Read the model definition and answer for the solid it produces. Units are mm, in the model's axes. Face numbers are marked on the shaded views. A direction names the side the tool comes from. Round coordinates to 2 decimals unless told otherwise and drop trailing zeros. Order: outer loops, then holes, each group sorted by start corner. A loop starts at its lowest first (then second) coordinate and runs counter-clockwise, first axis right, second up.
Autodesk Inventor part; units mm, degrees
ref_plane "YZ Plane" through (0, 0, 0) normal (1, 0, 0) x (0, 1, 0)
ref_plane "XZ Plane" through (0, 0, 0) normal (0, 1, 0) x (-1, 0, 0)
ref_plane "XY Plane" through (0, 0, 0) normal (0, 0, 1) x (1, 0, 0)
sketch "Sketch1" plane through (0, 0, 0) normal (0, 0, 1) x (1, 0, 0)
  circle A0 centre (0, 0) radius 42.5
  dimension "d0" = 85
extrude "Extrusion1" add sketch "Sketch1" along normal blind 5
sketch "Sketch2" plane through (0, 0, 5) normal (0, 0, 1) x (1, 0, 0)
  circle A0 centre (0, 0) radius 13
  dimension "d3" = 26
extrude "Extrusion2" add sketch "Sketch2" along normal blind 20
sketch "Sketch3" plane through (0, 0, 25) normal (0, 0, 1) x (1, 0, 0)
  circle A0 centre (0, 0) radius 42.5
  dimension "d6" = 85
extrude "Extrusion3" add sketch "Sketch3" along normal blind 5
sketch "Sketch4" plane through (0, 0, 0) normal (0, 0, -1) x (-1, 0, 0)
  circle A0 centre (0, 0) radius 11
  dimension "d9" = 22
extrude "Extrusion4" cut sketch "Sketch4" against normal through all
properties part number "wire_spool_holder"
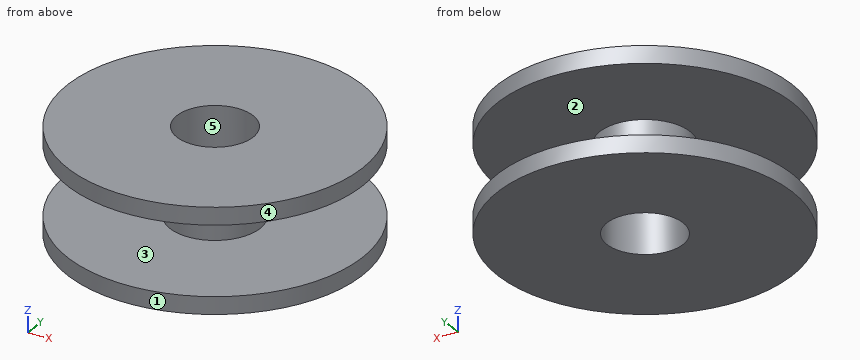
Q1. For the marked faces 1 and 2, determine the directions among +Z, -Z, +X, -X, +Y, -Y from which every point of the face is accessible in a straight line to the end or side of a thin tool.
Outcome:
face 1: +Z, -Z
face 2: none
Q2. A cutting plane is placed at A-A, the plane x = -25.5. Give the vertices of the cut face in (y, z).
Outcome:
outline: (-34, 0) - (34, 0) - (34, 5) - (-34, 5) - close; (-34, 25) - (34, 25) - (34, 30) - (-34, 30) - close
Q3. Straight lines are drawn through the part: probe 1 along Z at (x, y) = (-16, -11.5); probe 2 along Y at (x, z) = (0, 7.75); probe 3 along Y at (x, z) = (1, 26.75). For each, find the intervals that lie inside material, in ascending order.
Outcome:
probe 1: z = 0 to 5, 25 to 30
probe 2: y = -13 to -11, 11 to 13
probe 3: y = -42.49 to -10.95, 10.95 to 42.49
Q4. For a pull along X with two mould halves and no side action, classify the marked faces 3, 4 and 5 as released by +X, released by -X, zero draft, split by the parting line, or undercut.
Outcome:
face 3: zero draft
face 4: split by the parting line
face 5: undercut
Q5. Flat-ended cylindrical pins translate along their axes: pin 1 (1 mm diameter, centred on y = 11.5, z = 6.5, fed in from -X); pin 2 (4 mm diameter, centred on y = -24, z = 8, fed in from +X); pin 3 (12 mm diameter, centred on y = 34, z = 7.5, fed in from +X); pin 4 (5 mm diameter, centred on y = -34, z = 25, fed in from -X). Find the tip coordinate at first contact, or state that the pin passes through.
Outcome:
pin 1: stops at x = -6.93
pin 2: passes through
pin 3: stops at x = 31.49
pin 4: stops at x = -28.53
Q6. A cutting plane is placed at C-C, the plane z = 7.25. Give the vertices of the cut face in (x, y).
Outcome:
outline: circle Ø26 at (0, 0); hole circle Ø22 at (0, 0)
Q7. A cutting plane is placed at B-B, the plane y = 0. Give the vertices of the cut face in (x, z), plus the area to 3 significant figures.
Outcome:
outline: (-42.5, 0) - (-11, 0) - (-11, 30) - (-42.5, 30) - (-42.5, 25) - (-13, 25) - (-13, 5) - (-42.5, 5) - close; (11, 0) - (42.5, 0) - (42.5, 5) - (13, 5) - (13, 25) - (42.5, 25) - (42.5, 30) - (11, 30) - close
area: 710 mm2
